```python
from build123d import *

# Parameters (mm, degrees)
SKETCH1_R           = 1.054
BOSS_EXTRUDE1_DEPTH = 3
SKETCH3_R           = 1.1
BOSS_EXTRUDE2_DEPTH = 3
CUT_EXTRUDE1_DEPTH  = 23.736281859
SKETCH4_R           = 1.5
BOSS_EXTRUDE3_DEPTH = 1
FILLET1_R           = 1


with BuildPart() as part:
    # Sketch1 → Boss-Extrude1 (new body)
    with BuildSketch(Plane(origin=(0, 0, 0), x_dir=(1, 0, 0), z_dir=(0, 1, 0))):
        with BuildLine():
            Line((0, 0), (9.035898385, 0))
            ThreePointArc((9.035898385, 0), (10.767949192, 1), (10.767949192, 3))
            Line((10.767949192, 3), (1.732050808, 18.650635095))
            ThreePointArc((1.732050808, 18.650635095), (0, 19.650635095), (-1.732050808, 18.650635095))
            Line((-1.732050808, 18.650635095), (-10.767949192, 3))
            ThreePointArc((-10.767949192, 3), (-10.767949192, 1), (-9.035898385, 0))
            Line((-9.035898385, 0), (0, 0))
        make_face()
        with Locations(Location((0, 17.650635095, 0), (0, 0, 270))):
            Circle(SKETCH1_R, mode=Mode.SUBTRACT)
        with Locations(Location((-9.035898385, 2, 0), (0, 0, 270))):
            Circle(SKETCH1_R, mode=Mode.SUBTRACT)
        with Locations(Location((9.035898385, 2, 0), (0, 0, 270))):
            Circle(SKETCH1_R, mode=Mode.SUBTRACT)
    extrude(amount=BOSS_EXTRUDE1_DEPTH)

    # Sketch3 → Boss-Extrude2 (add)
    with BuildSketch(Plane(origin=(0, 3, 0), x_dir=(1, 0, 0), z_dir=(0, 1, 0))):
        with BuildLine():
            Line((-9.526279442, 14.216878365), (9.526279442, 14.216878365))
            ThreePointArc((9.526279442, 14.216878365), (10.825317547, 13.466878365), (10.825317547, 11.966878365))
            Line((10.825317547, 11.966878365), (1.299038106, -4.533121635))
            ThreePointArc((1.299038106, -4.533121635), (0, -5.283121635), (-1.299038106, -4.533121635))
            Line((-1.299038106, -4.533121635), (-10.825317547, 11.966878365))
            ThreePointArc((-10.825317547, 11.966878365), (-10.825317547, 13.466878365), (-9.526279442, 14.216878365))
        make_face()
        with Locations(Location((0, -3.783121635, 0), (0, 0, 270))):
            Circle(SKETCH3_R, mode=Mode.SUBTRACT)
        with Locations(Location((-9.526279442, 12.716878365, 0), (0, 0, 270))):
            Circle(SKETCH3_R, mode=Mode.SUBTRACT)
        with Locations(Location((9.526279442, 12.716878365, 0), (0, 0, 270))):
            Circle(SKETCH3_R, mode=Mode.SUBTRACT)
    extrude(amount=-BOSS_EXTRUDE2_DEPTH)

    # Sketch2 → Cut-Extrude1 (cut, through all)
    with BuildSketch(Plane(origin=(0, 3, 0), x_dir=(1, 0, 0), z_dir=(0, 1, 0))):
        with BuildLine():
            Line((-1, 15.918584287), (-2.848505776, 12.716878365))
            Line((-2.848505776, 12.716878365), (-7.526279442, 12.716878365))
            ThreePointArc((-7.526279442, 12.716878365), (-7.794228634, 11.716878365), (-8.526279442, 10.984827557))
            Line((-8.526279442, 10.984827557), (-6.187392609, 6.93375673))
            Line((-6.187392609, 6.93375673), (-8.035898385, 3.732050808))
            ThreePointArc((-8.035898385, 3.732050808), (-7.303847577, 3), (-7.035898385, 2))
            Line((-7.035898385, 2), (-3.338886833, 2))
            Line((-3.338886833, 2), (-1, -2.051070828))
            ThreePointArc((-1, -2.051070828), (0, -1.783121635), (1, -2.051070828))
            Line((1, -2.051070828), (3.338886833, 2))
            Line((3.338886833, 2), (7.035898385, 2))
            ThreePointArc((7.035898385, 2), (7.303847577, 3), (8.035898385, 3.732050808))
            Line((8.035898385, 3.732050808), (6.187392609, 6.93375673))
            Line((6.187392609, 6.93375673), (8.526279442, 10.984827557))
            ThreePointArc((8.526279442, 10.984827557), (7.794228634, 11.716878365), (7.526279442, 12.716878365))
            Line((7.526279442, 12.716878365), (2.848505776, 12.716878365))
            Line((2.848505776, 12.716878365), (1, 15.918584287))
            ThreePointArc((1, 15.918584287), (0, 15.650635095), (-1, 15.918584287))
        make_face()
    extrude(amount=-CUT_EXTRUDE1_DEPTH, mode=Mode.SUBTRACT)

    # Sketch4 → Boss-Extrude3 (add)
    with BuildSketch(Plane.XZ):
        with Locations(Location((0, 3.783121635, 0), (0, 0, 30))):
            Circle(SKETCH4_R)
        with Locations(Location((9.526279442, -12.716878365, 0), (0, 0, 270))):
            Circle(SKETCH4_R)
        with Locations(Location((-9.526279442, -12.716878365, 0), (0, 0, 270))):
            Circle(SKETCH4_R)
    extrude(amount=BOSS_EXTRUDE3_DEPTH)

    # Fillet1
    fillet1_edges = [part.edges().sort_by_distance(p)[0] for p in [
        (-1.299038106, -1, 3.033121635),
        (9.526279442, -1, -11.216878365),
        (-9.526279442, -1, -11.216878365),
    ]]
    fillet(fillet1_edges, radius=FILLET1_R - 0.0001)  # a hair under: the kernel refuses the full size


solid = part.part
```
Can you work these out from the model? Positions are in its coordinate system, mm. A direction names the side the tool comes from. Round coordinates to 2 decimals unless told otherwise and drop trailing zeros. Order: outer loops, then holes, each group sorted by start corner. A loop starts at its lowest first (then second) coordinate and runs counter-clockwise, first axis right, second up.
(1) If we section it at B-B (z = -17.75): Please give me the cut outline in (x, y), plus the area to 3 significant figures.
Results are:
outline: (-2.25, 0) - (-1.05, 0) - (-1.05, 3) - (-2.25, 3) - close; (1.05, 0) - (2.25, 0) - (2.25, 3) - (1.05, 3) - close
area: 7.22 mm2
(2) We'd pull the mould along Z, two halves only. Please class faces 6 (the face through (-8.15, 1.48, -1.43)), 7 (the face through (6, 1, 0)), 8 (the face through (7, 2, -14.217)), 9 (the face through (-7.31, 1.52, -3.01)): +Z half, -Z half, draft (parallel to the pull), parting line (faces both ways), or undercut.
Results are:
face 6: undercut
face 7: +Z half
face 8: -Z half
face 9: undercut
(3) I'm going to push flat-ended pins straight in: pin 1 (1.3 mm diameter, centred on x = 9.04, z = -2, fed in from +Y); pin 2 (0.9 mm diameter, centred on x = 7.5, y = 1, fed in from +Z); pin 3 (2.5 mm diameter, centred on x = -9.04, z = -2, fed in from -Y); pin 4 (0.9 mm diameter, centred on x = -6.5, y = 2, fed in from -Z). Where does each tip first touch, or does it pass through?
Results are:
pin 1: passes through
pin 2: stops at z = 0
pin 3: stops at y = 0
pin 4: stops at z = -14.22
(4) If we section it at C-C (x = 0): Count the separate pieces of the cut face and the enclosed holes in it, plus the area to 3 significant figures.
Results are:
separate pieces: 3
enclosed holes: 0
area: 12.1 mm2
(5) If I drill on L1, parallel to Z at x = 5.25, y = 1.15; L2, parallel to Z at x = -0.5, y = 0.25; L3, parallel to X at y = 0.3, z = -12.5, over which ranges is the centre line in solid material (lowest first)?
Results are:
L1: z = -14.22 to -12.72, -2 to 0
L2: z = -19.59 to -18.58, -16.72 to -15.71, 1.85 to 2.8, 4.76 to 5.2
L3: x = -11.01 to -10.6, -8.45 to -7.54, 7.54 to 8.45, 10.6 to 11.01
(6) On a 3-axis mill with a long thin cutter (end or side, diameter ignored), from which of +Z, -Z, +X, -X, +Y, -Y can I reach the whole of each face in a straight line? I mean faces 1 (the face through (-9.5, 1.52, -9.67)), 2 (the face through (-7, 1, 0)), 3 (the face through (0.01, 1.52, -15.65)), 4 (the face through (9.5, 1.5, -5.2)), 5 (the face through (0.33, 1.521, 4.832)). Say none if no direction works.
Results are:
face 1: -X, +Y, -Y
face 2: +Z, -X, +Y, -Y
face 3: +Y, -Y
face 4: +X, +Y, -Y
face 5: +Y
(7) If we section it at A-A (x = 2.5): Please give me the cut outline in (y, z), plus the area to 3 significant figures.
Results are:
outline: (0, -17.32) - (3, -17.32) - (3, -13.32) - (0, -13.32) - close; (0, -0.55) - (3, -0.55) - (3, 2.45) - (0, 2.45) - close
area: 21.0 mm2
